Check sheet for the modelled part. Datum: model origin and axes. Units: mm. A direction names the side the tool comes from. Round coordinates to 2 decimals unless told otherwise and drop trailing zeros. Write each loop counter-clockwise with the first axis right and the second up, starting at its lowest first coordinate (ties: lowest second). Pieces come first, ordered by that corner, then holes. Notation, with made-up numbers: (84.25, 76.25) - (133.25, 76.25) arc R7 cw to (133.25, 80.25) - close; hole circle Ø6 at (46.5, 51). An arc over 180 degrees is marked (long way). Answer as a JSON object with one key per item and string values. Group by question number.
Item 1: Sectioned sample at C-C on y = -7.75. Record the boundary of the cut face in (x, z) (1 decimal), plus the area to 3 significant figures.
Item 2: Thickness scan on line 1 (X direction, y = -7.05, z = 0); line 2 (Z direction, x = 0, y = -1.6); line 3 (X direction, y = -7, z = 0). Record the ranges inside material, lowest first.
Item 3: Set-up check for faces 1 (the flat face through (0, 0, 0)), 2 (the cylindrical face through (-0.8, -8.03, 19.94)), 3 (the cylindrical face through (-12.9, -1.97, 0.09)): record each of +Z, -Z, +X, -X, +Y, -Y from which the full face is reachable in a straight line by a thin tool's end or side.
Item 4: Release check for a two-part mould opening along X. For faces 4 (the conical face through (-3.96, -0.63, 17.85)), 5 (the flat face through (0, -10, 0)), 6 (the flat face through (0, -4, 15)) record: pulls with the +X half, pulls with the -X half, needs draft (parallel to the pull), parting line crosses it, or undercut.
Item 5: Sectioned sample at A-A on y = -1. Record the boundary of the cut face in (x, z), plus the area to 3 significant figures.
Item 6: Gauge pin test, flat ends, axial feed: P1, Ø1.3, axis at x = -0.5, z = 15, coming from the +Y side; P2, Ø5, axis at x = 18, z = 0, coming from the +Y side; P3, Ø1, axis at x = -1, y = -7.5, coming from the +Z side; P4, Ø1.5, axis at x = 17, z = 14.5, coming from the +Y side. Record the tip position at first contact, or that the pin passes through.
Item 7: Sectioned sample at B-B on y = -5.25. Record the boundary of the cut face in (x, z) (1 decimal).
```python
from build123d import *

# Parameters (mm, degrees)
SKETCH_26_R         = 2.1
CUT_EXTRUDE_2_DEPTH = 4
SKETCH_36_R         = 2.1
CUT_EXTRUDE_3_DEPTH = 4


with BuildPart() as part:
    # 草图8 → 旋转1 (revolve)
    with BuildSketch(Plane(origin=(0, 0, 0), x_dir=(-1, 0, 0), z_dir=(0, 0, -1))):
        Polygon((0, 0), (-18, 0), (-22.5, -10), (0, -10), align=None)
    revolve(axis=Axis((0, -10, 0), (0, 1, 0)))

    # 草图26 → 切除-拉伸2 (cut)
    with BuildSketch(Plane(origin=(0, -10, 0), x_dir=(1, 0, 0), z_dir=(0, 1, 0))):
        with Locations(Location((18, 0, 0), (0, 0, 270))):
            Circle(SKETCH_26_R)
        with Locations(Location((0, -18, 0), (0, 0, 270))):
            Circle(SKETCH_26_R)
        with Locations(Location((0, 18, 0), (0, 0, 270))):
            Circle(SKETCH_26_R)
        with Locations(Location((-18, 0, 0), (0, 0, 270))):
            Circle(SKETCH_26_R)
    extrude(amount=CUT_EXTRUDE_2_DEPTH, mode=Mode.SUBTRACT)

    # 草图36 → 切除-拉伸3 (cut)
    with BuildSketch(Plane(origin=(0, 0, 0), x_dir=(1, 0, 0), z_dir=(0, 1, 0))):
        with Locations(Location((0, 15, 0), (0, 0, 180))):
            Circle(SKETCH_36_R)
        with Locations(Location((15, 0, 0), (0, 0, 180))):
            Circle(SKETCH_36_R)
        with Locations(Location((0, -15, 0), (0, 0, 180))):
            Circle(SKETCH_36_R)
        with Locations(Location((-15, 0, 0), (0, 0, 180))):
            Circle(SKETCH_36_R)
    extrude(amount=-CUT_EXTRUDE_3_DEPTH, mode=Mode.SUBTRACT)


solid = part.part
```
Completed:
{
 "1": {"outline": "circle Ø43 at (0, 0); hole circle Ø4.2 at (-18, 0); hole circle Ø4.2 at (0, -18); hole circle Ø4.2 at (0, 18); hole circle Ø4.2 at (18, 0)", "area": "1,400 mm²"},
 "2": {"line 1": "-21.17 to -20.1, -15.9 to 15.9, 20.1 to 21.17", "line 2": "-18.72 to -17.1, -12.9 to 12.9, 17.1 to 18.72", "line 3": "-21.15 to -20.1, -15.9 to 15.9, 20.1 to 21.15"},
 "3": {"face 1": "+Z, -Z, +X, -X, +Y", "face 2": "-Y", "face 3": "+Y"},
 "4": {"face 4": "parting line crosses it", "face 5": "needs draft", "face 6": "undercut"},
 "5": {"outline": "circle Ø36.9 at (0, 0); hole circle Ø4.2 at (-15, 0); hole circle Ø4.2 at (0, -15); hole circle Ø4.2 at (0, 15); hole circle Ø4.2 at (15, 0)", "area": "1,010 mm²"},
 "6": {"P1": "y = -4", "P2": "y = 0", "P3": "z = 21.58", "P4": "y = -7.99"},
 "7": {"outline": "circle Ø40.7 at (0, 0)"}
}
